```python
from build123d import *

# Parameters (mm, degrees)
F0_W     = 1.5
F0_H     = 1.5
F1_DEPTH = 2


with BuildPart() as f1:
    # F0 (on Top) → F1 (new body)
    with BuildSketch(Plane.XY):
        Polygon((26.65, -10.914245), (26.65, 29.085755), (25.45, 29.085755), (23.45, 29.085755), (6.35, 29.085755), (6.35, 24.085755), (-6.65, 24.085755), (-6.65, 29.085755), (-23.45, 29.085755), (-25.45, 29.085755), (-26.65, 29.085755), (-26.65, -20.414245), (11.65, -20.414245), (11.65, -10.914245), align=None)
        with Locations((-24.45, -17.064245)):
            Rectangle(F0_W, F0_H, mode=Mode.SUBTRACT)
        with Locations((-24.45, -14.564245)):
            Rectangle(F0_W, F0_H, mode=Mode.SUBTRACT)
        with Locations((-24.45, -12.064245)):
            Rectangle(F0_W, F0_H, mode=Mode.SUBTRACT)
        with Locations((-24.45, -9.564245)):
            Rectangle(F0_W, F0_H, mode=Mode.SUBTRACT)
        with Locations((-24.45, -7.064245)):
            Rectangle(F0_W, F0_H, mode=Mode.SUBTRACT)
        with Locations((-24.45, -4.564245)):
            Rectangle(F0_W, F0_H, mode=Mode.SUBTRACT)
        with Locations((-24.45, -2.064245)):
            Rectangle(F0_W, F0_H, mode=Mode.SUBTRACT)
        with Locations((-24.45, 0.435755)):
            Rectangle(F0_W, F0_H, mode=Mode.SUBTRACT)
        with Locations((-24.45, 2.935755)):
            Rectangle(F0_W, F0_H, mode=Mode.SUBTRACT)
        with Locations((24.45, -8.064245)):
            Rectangle(F0_W, F0_H, mode=Mode.SUBTRACT)
        with Locations((24.45, -5.564245)):
            Rectangle(F0_W, F0_H, mode=Mode.SUBTRACT)
        with Locations((24.45, -3.064245)):
            Rectangle(F0_W, F0_H, mode=Mode.SUBTRACT)
        with Locations((24.45, -0.564245)):
            Rectangle(F0_W, F0_H, mode=Mode.SUBTRACT)
        with Locations((24.45, 1.935755)):
            Rectangle(F0_W, F0_H, mode=Mode.SUBTRACT)
        with Locations((-24.45, 5.435755)):
            Rectangle(F0_W, F0_H, mode=Mode.SUBTRACT)
        with Locations((-24.45, 10.085755)):
            Rectangle(F0_W, F0_H, mode=Mode.SUBTRACT)
        with Locations((-24.45, 12.585755)):
            Rectangle(F0_W, F0_H, mode=Mode.SUBTRACT)
        with Locations((-24.45, 15.085755)):
            Rectangle(F0_W, F0_H, mode=Mode.SUBTRACT)
        with Locations((-24.45, 17.585755)):
            Rectangle(F0_W, F0_H, mode=Mode.SUBTRACT)
        with Locations((-24.45, 20.085755)):
            Rectangle(F0_W, F0_H, mode=Mode.SUBTRACT)
        with Locations((-24.45, 22.585755)):
            Rectangle(F0_W, F0_H, mode=Mode.SUBTRACT)
        with Locations((-24.45, 25.085755)):
            Rectangle(F0_W, F0_H, mode=Mode.SUBTRACT)
        with Locations((-24.45, 27.585755)):
            Rectangle(F0_W, F0_H, mode=Mode.SUBTRACT)
        with Locations((24.45, 4.435755)):
            Rectangle(F0_W, F0_H, mode=Mode.SUBTRACT)
        with Locations((24.45, 6.935755)):
            Rectangle(F0_W, F0_H, mode=Mode.SUBTRACT)
        with Locations((24.45, 9.435755)):
            Rectangle(F0_W, F0_H, mode=Mode.SUBTRACT)
        with Locations((24.45, 15.085755)):
            Rectangle(F0_W, F0_H, mode=Mode.SUBTRACT)
        with Locations((24.45, 17.585755)):
            Rectangle(F0_W, F0_H, mode=Mode.SUBTRACT)
        with Locations((24.45, 20.085755)):
            Rectangle(F0_W, F0_H, mode=Mode.SUBTRACT)
        with Locations((24.45, 22.585755)):
            Rectangle(F0_W, F0_H, mode=Mode.SUBTRACT)
        with Locations((24.45, 25.085755)):
            Rectangle(F0_W, F0_H, mode=Mode.SUBTRACT)
        Polygon((25.2, 28.085755), (25.2, 26.835755), (23.7, 26.835755), (23.7, 28.335755), (25.2, 28.335755), align=None, mode=Mode.SUBTRACT)
    extrude(amount=F1_DEPTH)


solid = f1.part
```
The model under review builds one solid part; all positions refer to its coordinate system, in mm. Round coordinates to 2 decimals unless told otherwise and drop trailing zeros. Loops run counter-clockwise (first coordinate to the right, second up) from the corner with the lowest first, then second, coordinate; pieces in that order, holes last. Notation, with made-up numbers: (-10.5, 19) -> (-0.5, 19) arc R22 ccw to (-0.5, 33) -> close; hole circle Ø1 at (39, 77.5). An arc over 180 degrees is marked (long way). Answer as a JSON object with one key per item and string values. Group by question number.
1) We need section A-A on z = 0.3. Give the number of separate pieces and of enclosed holes in the cut face, then the cut area to 3 significant figures.
2) We need section B-B on x = 0. Write out the cut boundary in (y, z).
3) For pin 1 Ø1.2 at (y, z) = (-12, 1) entering from +X, flat-tipped, find the tip position at first contact; note if it passes through.
4) We need section C-C on x = 19.5. Write out the cut boundary in (y, z), then the cut area to 3 significant figures.
5) For line 1 (X direction, y = 18, z = 1.4); line 2 (X direction, y = -3.5, z = 0.4); line 3 (X direction, y = 12.5, z = 0.75), list the stretches that pass through material, from the lowest coordinate up. Write a range as [from, to].
6) Mouldability with a two-part tool opening along Y and no side actions: class faces 1 (the face through (-23.7, -7, 1)), 2 (the face through (24, 18.336, 1)), 3 (the face through (11.65, -16, 1)) as released by +Y, released by -Y, zero draft, split by the parting line, or undercut.
Result set:
{
 "1": {"separate pieces": "1", "enclosed holes": "32", "area": "2,360 mm²"},
 "2": {"outline": "(-20.41, 0) -> (24.09, 0) -> (24.09, 2) -> (-20.41, 2) -> close"},
 "3": {"pin 1": "x = 11.65"},
 "4": {"outline": "(-10.91, 0) -> (29.09, 0) -> (29.09, 2) -> (-10.91, 2) -> close", "area": "80.0 mm²"},
 "5": {"line 1": "[-26.65, -25.2], [-23.7, 23.7], [25.2, 26.65]", "line 2": "[-26.65, 23.7], [25.2, 26.65]", "line 3": "[-26.65, -25.2], [-23.7, 26.65]"},
 "6": {"face 1": "undercut", "face 2": "undercut", "face 3": "zero draft"}
}
